from build123d import *

# Parameters (mm, degrees)
SKETCH1_R           = 4.2
BOSS_EXTRUDE1_DEPTH = 5
FILLET1_R           = 10
FILLET2_R           = 6
SKETCH2_W           = 42
SKETCH2_H           = 46
SKETCH2_R           = 11.5
SKETCH2_R_2         = 1.75
BOSS_EXTRUDE2_DEPTH = 4
CUT_EXTRUDE1_REACH  = 89.139
CUT_EXTRUDE1_START  = -1
SKETCH3_R           = 3
CUT_EXTRUDE2_REACH  = 90.34
SKETCH4_R           = 1.75
SKETCH5_R           = 2.1
CUT_EXTRUDE3_DEPTH  = 4
BOSS_EXTRUDE3_START = -2
BOSS_EXTRUDE3_DEPTH = 3
FILLET3_R           = 2
FILLET4_R           = 3
SKETCH7_R           = 1.75
CUT_EXTRUDE4_DEPTH  = 81.398748245
SKETCH8_R           = 2.1
CUT_EXTRUDE5_DEPTH  = 4
CHAMFER1_SIZE       = 0.5


with BuildPart() as part:
    # Sketch1 → Boss-Extrude1 (new, symmetric)
    with BuildSketch(Plane.XY):
        with BuildLine():
            Line((-52, 25), (52, 25))
            Line((52, 25), (52, 15.565713714))
            ThreePointArc((52, 15.565713714), (46, 1.282856857), (52, -13))
            Line((52, -13), (52, -25))
            Line((52, -25), (30, -25))
            ThreePointArc((30, -25), (0, -19.161984871), (-30, -25))
            Line((-30, -25), (-52, -25))
            Line((-52, -25), (-52, -13))
            ThreePointArc((-52, -13), (-46, 1.282856857), (-52, 15.565713714))
            Line((-52, 15.565713714), (-52, 25))
        make_face()
        with Locations((0, -11)):
            Circle(SKETCH1_R, mode=Mode.SUBTRACT)
        with Locations((-32, 7)):
            Circle(SKETCH1_R, mode=Mode.SUBTRACT)
        with Locations((32, 7)):
            Circle(SKETCH1_R, mode=Mode.SUBTRACT)
        with BuildLine():
            Line((-9.5, 21), (9.5, 21))
            ThreePointArc((9.5, 21), (10.560660172, 20.560660172), (11, 19.5))
            Line((11, 19.5), (11, 2.5))
            ThreePointArc((11, 2.5), (10.560660172, 1.439339828), (9.5, 1))
            Line((9.5, 1), (-9.5, 1))
            ThreePointArc((-9.5, 1), (-10.560660172, 1.439339828), (-11, 2.5))
            Line((-11, 2.5), (-11, 19.5))
            ThreePointArc((-11, 19.5), (-10.560660172, 20.560660172), (-9.5, 21))
        make_face(mode=Mode.SUBTRACT)
    extrude(amount=BOSS_EXTRUDE1_DEPTH, both=True)

    # Fillet1
    # the kernel refuses this fillet: 10 mm, written as the material it takes off along each edge
    with BuildSketch(Plane(origin=(52, 15.565713714, 14.292857857), x_dir=(-0.6589710561597435, -0.7521682970876347, 0), z_dir=(0, 0, -1))) as fillet1_piece_1:
        with BuildLine():
            CenterArc((3.793793334, 9.971172714), FILLET1_R, 228.778553177, 36.869897646)
            Line((-2.795917228, 2.449489743), (0, 0))
            ThreePointArc((0, 0), (1.517517334, 0.057654573), (3.035034667, 0))
        make_face()
    extrude(amount=28.585715715, mode=Mode.SUBTRACT)
    with BuildSketch(Plane(origin=(52, -13, 14.292857857), x_dir=(0, -1, 0), z_dir=(0, 0, -1)), Plane(origin=(-52, -13, -14.292857857), x_dir=(0, -1, 0), z_dir=(0, 0, 1))) as fillet1_piece_2:
        with BuildLine():
            CenterArc((3.717143143, 10), FILLET1_R, 233.130102354, 36.869897646)
            ThreePointArc((-2.282856857, 2), (-1.103435734, 1.043365942), (0, 0))
            Line((0, 0), (3.717143143, 0))
        make_face()
    extrude(amount=28.585715715, mode=Mode.SUBTRACT)
    with BuildSketch(Plane(origin=(52, -25, 30), x_dir=(-1, 0, 0), z_dir=(0, 0, -1))) as fillet1_piece_3:
        with BuildLine():
            CenterArc((FILLET1_R, FILLET1_R), FILLET1_R, 180, 90)
            Line((0, FILLET1_R), (0, 0))
            Line((0, 0), (FILLET1_R, 0))
        make_face()
    extrude(amount=60, mode=Mode.SUBTRACT)
    with BuildSketch(Plane(origin=(30, -25, 9.716697693), x_dir=(-0.931136532102541, 0.3646707536724787, 0), z_dir=(0, 0, -1))) as fillet1_piece_4:
        with BuildLine():
            CenterArc((1.889951723, 9.999382002), FILLET1_R, 248.612678269, 20.750330625)
            Line((-1.756755813, 0.688016681), (0, 0))
            ThreePointArc((0, 0), (0.889389046, 0.004943983), (1.778778093, 0))
        make_face()
    extrude(amount=19.433395387, mode=Mode.SUBTRACT)
    with BuildSketch(Plane(origin=(-30, -25, 9.716697693), x_dir=(-1, 0, 0), z_dir=(0, 0, -1))) as fillet1_piece_5:
        with BuildLine():
            CenterArc((1.886679077, 10), FILLET1_R, 249.249669375, 20.750330625)
            ThreePointArc((-1.656285265, 0.648668348), (-0.826339706, 0.328937697), (0, 0))
            Line((0, 0), (1.886679077, 0))
        make_face()
    extrude(amount=19.433395387, mode=Mode.SUBTRACT)
    with BuildSketch(Plane(origin=(-52, -25, -30), x_dir=(0, 1, 0), z_dir=(0, 0, 1))) as fillet1_piece_6:
        with BuildLine():
            CenterArc((FILLET1_R, -FILLET1_R), FILLET1_R, 90, 90)
            Line((0, -FILLET1_R), (0, 0))
            Line((0, 0), (FILLET1_R, 0))
        make_face()
    extrude(amount=60, mode=Mode.SUBTRACT)
    with BuildSketch(Plane(origin=(-52, 15.565713714, -14.292857857), x_dir=(0, 1, 0), z_dir=(0, 0, 1))) as fillet1_piece_7:
        with BuildLine():
            CenterArc((3.717143143, -10), FILLET1_R, 90, 36.869897646)
            ThreePointArc((-2.282856857, -2), (-1.103435734, -1.043365942), (0, 0))
            Line((0, 0), (3.717143143, 0))
        make_face()
    extrude(amount=28.585715715, mode=Mode.SUBTRACT)

    # Fillet2
    fillet2_edges = [part.edges().sort_by_distance(p)[0] for p in [
        (52, 25, 0),
        (-52, 25, 0),
    ]]
    fillet(fillet2_edges, radius=FILLET2_R)

    # Sketch2 → Boss-Extrude2 (add)
    with BuildSketch(Plane(origin=(0, 25, -30), x_dir=(-1, 0, 0), z_dir=(0, 1, 0))):
        with Locations((0, 2)):
            Rectangle(SKETCH2_W, SKETCH2_H)
        with Locations(Location((0, 1, 0), (0, 0, 90))):
            Circle(SKETCH2_R, mode=Mode.SUBTRACT)
        with Locations(Location((15.5, 16.5, 0), (0, 0, 90))):
            Circle(SKETCH2_R_2, mode=Mode.SUBTRACT)
        with Locations(Location((-15.5, 16.5, 0), (0, 0, 90))):
            Circle(SKETCH2_R_2, mode=Mode.SUBTRACT)
        with Locations(Location((-15.5, -14.5, 0), (0, 0, 90))):
            Circle(SKETCH2_R_2, mode=Mode.SUBTRACT)
        with Locations(Location((15.5, -14.5, 0), (0, 0, 90))):
            Circle(SKETCH2_R_2, mode=Mode.SUBTRACT)
    extrude(amount=-BOSS_EXTRUDE2_DEPTH)

    # Sketch3 → Cut-Extrude1 (cut, up to next)
    with BuildSketch(Plane.XZ.offset(-21).offset(CUT_EXTRUDE1_START), mode=Mode.PRIVATE) as cut_extrude1_sk1:
        with Locations(Location((-15.5, -44.5, 0), (0, 0, 270))):
            Circle(SKETCH3_R)
    cut_extrude1_tool1 = extrude(cut_extrude1_sk1.sketch, amount=CUT_EXTRUDE1_REACH, mode=Mode.PRIVATE) & part.part
    # Sketch3 → Cut-Extrude1 (cut, up to next)
    with BuildSketch(Plane.XZ.offset(-21).offset(CUT_EXTRUDE1_START), mode=Mode.PRIVATE) as cut_extrude1_sk2:
        with Locations(Location((15.5, -44.5, 0), (0, 0, 270))):
            Circle(SKETCH3_R)
    cut_extrude1_tool2 = extrude(cut_extrude1_sk2.sketch, amount=CUT_EXTRUDE1_REACH, mode=Mode.PRIVATE) & part.part
    # Sketch3 → Cut-Extrude1 (cut, up to next)
    with BuildSketch(Plane.XZ.offset(-21).offset(CUT_EXTRUDE1_START), mode=Mode.PRIVATE) as cut_extrude1_sk3:
        with Locations(Location((15.5, -13.5, 0), (0, 0, 270))):
            Circle(SKETCH3_R)
    cut_extrude1_tool3 = extrude(cut_extrude1_sk3.sketch, amount=CUT_EXTRUDE1_REACH, mode=Mode.PRIVATE) & part.part
    # Sketch3 → Cut-Extrude1 (cut, up to next)
    with BuildSketch(Plane.XZ.offset(-21).offset(CUT_EXTRUDE1_START), mode=Mode.PRIVATE) as cut_extrude1_sk4:
        with Locations(Location((-15.5, -13.5, 0), (0, 0, 270))):
            Circle(SKETCH3_R)
    cut_extrude1_tool4 = extrude(cut_extrude1_sk4.sketch, amount=CUT_EXTRUDE1_REACH, mode=Mode.PRIVATE) & part.part
    add(cut_extrude1_tool1.solids().sort_by_distance((-15.5, 22, -44.5))[0], mode=Mode.SUBTRACT)
    add(cut_extrude1_tool2.solids().sort_by_distance((15.5, 22, -44.5))[0], mode=Mode.SUBTRACT)
    add(cut_extrude1_tool3.solids().sort_by_distance((15.5, 22, -13.5))[0], mode=Mode.SUBTRACT)
    add(cut_extrude1_tool4.solids().sort_by_distance((-15.5, 22, -13.5))[0], mode=Mode.SUBTRACT)

    # Sketch4 → Cut-Extrude2 (cut, up to next)
    with BuildSketch(Plane(origin=(0, 25, 0), x_dir=(1, 0, 0), z_dir=(0, 1, 0)), mode=Mode.PRIVATE) as cut_extrude2_sk1:
        with Locations(Location((-32, 0, 0), (0, 0, 270))):
            Circle(SKETCH4_R)
    cut_extrude2_tool1 = extrude(cut_extrude2_sk1.sketch, amount=-CUT_EXTRUDE2_REACH, mode=Mode.PRIVATE) & part.part
    # Sketch4 → Cut-Extrude2 (cut, up to next)
    with BuildSketch(Plane(origin=(0, 25, 0), x_dir=(1, 0, 0), z_dir=(0, 1, 0)), mode=Mode.PRIVATE) as cut_extrude2_sk2:
        with Locations(Location((32, 0, 0), (0, 0, 270))):
            Circle(SKETCH4_R)
    cut_extrude2_tool2 = extrude(cut_extrude2_sk2.sketch, amount=-CUT_EXTRUDE2_REACH, mode=Mode.PRIVATE) & part.part
    add(cut_extrude2_tool1.solids().sort_by_distance((-32, 25, 0))[0], mode=Mode.SUBTRACT)
    add(cut_extrude2_tool2.solids().sort_by_distance((32, 25, 0))[0], mode=Mode.SUBTRACT)

    # Sketch5 → Cut-Extrude3 (cut)
    with BuildSketch(Plane(origin=(0, 25, 0), x_dir=(1, 0, 0), z_dir=(0, 1, 0))):
        with Locations(Location((-32, 0, 0), (0, 0, 270))):
            Circle(SKETCH5_R)
        with Locations(Location((32, 0, 0), (0, 0, 270))):
            Circle(SKETCH5_R)
    extrude(amount=-CUT_EXTRUDE3_DEPTH, mode=Mode.SUBTRACT)

    # Sketch6 → Boss-Extrude3 (add)
    with BuildSketch(Plane(origin=(21, 0, 0), x_dir=(0, 0, -1), z_dir=(1, 0, 0)).offset(BOSS_EXTRUDE3_START)):
        Polygon((51, 25), (5, 25), (5, 5), (51, 21), align=None)
    boss_extrude3 = extrude(amount=BOSS_EXTRUDE3_DEPTH)

    # Mirror1: Boss-Extrude3 across plane
    add(boss_extrude3.mirror(Plane(origin=(0, 0, 0), x_dir=(0, 0, 1), z_dir=(1, 0, 0))))

    # Fillet3
    fillet3_edges = [part.edges().sort_by_distance(p)[0] for p in [
        (-14.25, 21, -5),
        (14.25, 21, -5),
    ]]
    fillet(fillet3_edges, radius=FILLET3_R)

    # Fillet4
    fillet4_edges = [part.edges().sort_by_distance(p)[0] for p in [
        (22, 15, -5),
        (-22, 15, -5),
        (-22, 23, -51),
        (22, 23, -51),
    ]]
    fillet(fillet4_edges, radius=FILLET4_R)

    # Sketch7 → Cut-Extrude4 (cut, through all)
    with BuildSketch(Plane.XY.offset(5)):
        with Locations((-20, -9)):
            Circle(SKETCH7_R)
        with Locations((20, -9)):
            Circle(SKETCH7_R)
    extrude(amount=-CUT_EXTRUDE4_DEPTH, mode=Mode.SUBTRACT)

    # Sketch8 → Cut-Extrude5 (cut)
    with BuildSketch(Plane.XY.offset(5)):
        with Locations((-20, -9)):
            Circle(SKETCH8_R)
        with Locations((20, -9)):
            Circle(SKETCH8_R)
    extrude(amount=-CUT_EXTRUDE5_DEPTH, mode=Mode.SUBTRACT)

    # Chamfer1
    # the kernel refuses this chamfer: 0.5 mm, written as the material it takes off along each edge
    with BuildSketch(Plane(origin=(-32, 21, 0), x_dir=(0, 0, 1), z_dir=(-1, 0, 0))) as chamfer1_piece_1_section:
        Polygon((1.75, -CHAMFER1_SIZE), (1.75 + CHAMFER1_SIZE, 0), (1.75, 0), align=None)
    chamfer1_piece_1 = revolve(axis=Axis((-32, 21, 0), (0, 1, 0)), mode=Mode.PRIVATE)
    chamfer1_piece_1 = chamfer1_piece_1 & Plane(origin=(-32, 20.675956313, 0), x_dir=(0, 0, 1), z_dir=(0, 1, 0)) * Cylinder(2.1, 9, mode=Mode.PRIVATE)
    add(chamfer1_piece_1, mode=Mode.SUBTRACT)
    with BuildSketch(Plane(origin=(32, 21, 0), x_dir=(0, 0, 1), z_dir=(-1, 0, 0))) as chamfer1_piece_2_section:
        Polygon((1.75, -CHAMFER1_SIZE), (1.75 + CHAMFER1_SIZE, 0), (1.75, 0), align=None)
    chamfer1_piece_2 = revolve(axis=Axis((32, 21, 0), (0, 1, 0)), mode=Mode.PRIVATE)
    chamfer1_piece_2 = chamfer1_piece_2 & Plane(origin=(32, 20.675956313, 0), x_dir=(0, 0, 1), z_dir=(0, 1, 0)) * Cylinder(2.1, 10, mode=Mode.PRIVATE)
    add(chamfer1_piece_2, mode=Mode.SUBTRACT)
    with BuildSketch(Plane(origin=(-20, -9, 1), x_dir=(1, 0, 0), z_dir=(0, -1, 0))) as chamfer1_piece_3_section:
        Polygon((1.75, -CHAMFER1_SIZE), (1.75 + CHAMFER1_SIZE, 0), (1.75, 0), align=None)
    chamfer1_piece_3 = revolve(axis=Axis((-20, -9, 1), (0, 0, 1)), mode=Mode.PRIVATE)
    chamfer1_piece_3 = chamfer1_piece_3 & Plane(origin=(-20, -9, 0.675956313), x_dir=(1, 0, 0), z_dir=(0, 0, 1)) * Cylinder(2.1, 9, mode=Mode.PRIVATE)
    add(chamfer1_piece_3, mode=Mode.SUBTRACT)
    with BuildSketch(Plane(origin=(20, -9, 1), x_dir=(1, 0, 0), z_dir=(0, -1, 0))) as chamfer1_piece_4_section:
        Polygon((1.75, -CHAMFER1_SIZE), (1.75 + CHAMFER1_SIZE, 0), (1.75, 0), align=None)
    chamfer1_piece_4 = revolve(axis=Axis((20, -9, 1), (0, 0, 1)), mode=Mode.PRIVATE)
    chamfer1_piece_4 = chamfer1_piece_4 & Plane(origin=(20, -9, 0.675956313), x_dir=(1, 0, 0), z_dir=(0, 0, 1)) * Cylinder(2.1, 9, mode=Mode.PRIVATE)
    add(chamfer1_piece_4, mode=Mode.SUBTRACT)


solid = part.part
The model under review builds one solid part; all positions refer to its coordinate system, in mm. A direction names the side the tool comes from. Round coordinates to 2 decimals unless told otherwise and drop trailing zeros. Write each loop counter-clockwise with the first axis right and the second up, starting at its lowest first coordinate (ties: lowest second). Pieces come first, ordered by that corner, then holes. Notation, with made-up numbers: M 27,20.25 L 52,20.25 A18 ccw 52,31.25 Z; hole C 84.25,72 d10. An arc over 180 degrees is marked long. Answer as CSV lines item,"result". Start each with the question number.
Q1. Wall thickness on line 1 along X through (y, z) = (23.95, -13.5); line 2 along X through (y, z) = (13.75, 0); line 3 along Z through (x, y) = (15.5, 21.2): over which ranges is each line inside the solid? List them lowest first.
Q2. The part is to be moulded in two halves that separate along Y. For faces 1 (the face through (-51.38, 15.82, -0.07)), 2 (the face through (22, 18, -23)), 3 (the face through (-17, 22, -15)), say which applies: +Y half, -Y half, draft (parallel to the pull), parting line (faces both ways), or undercut.
Q3. Consider section B-B, the plane y = -9. Give the boundary of the cut face in (x, z).
Q4. Consider section D-D, the plane x = -15.5. Give the boundary of the cut face in (y, z).
Q5. Tool access review of faces 4 (the face through (14.18, 20.43, -5.6)), 5 (the face through (22.9, 14.86, -5.86)): name each direction out of +Z, -Z, +X, -X, +Y, -Y from which nothing blocks a thin tool from reaching the whole face with its end or side.
Q6. Consider section A-A, the plane x = 0. Give the boundary of the cut face in (y, z), then the cut area to 3 significant figures.
Q7. Consider section C-C, the plane z = -23. Give the boundary of the cut face in (x, y), then the cut area to 3 significant figures.
Q8. Clearance check with flat-ended pins moving along their axes: P1, Ø13, axis at y = 11.5, z = -31, coming from the +X side; P2, Ø11, axis at x = 0, y = -11, coming from the -Z side; P3, Ø3, axis at y = 10.5, z = -18.5, coming from the -X side. State where each tip first meets the part, or that it passes through.
Result set:
1,line 1,"x = -22 to -17.25, -13.75 to 13.75, 17.25 to 22"
1,line 2,"x = -50.33 to -33.75, -30.25 to -11, 11 to 30.25, 33.75 to 50.33"
1,line 3,"z = -51 to -47.5, -41.5 to -16.5, -10.5 to 5"
2,face 1,"undercut"
2,face 2,"draft"
2,face 3,"-Y half"
3,outline,"M -48.85,-5 L -21.75,-5 L -21.75,0.5 L -22.1,0.85 L -22.1,5 L -48.85,5 Z; M -18.25,-5 L -3.69,-5 L -3.69,5 L -17.9,5 L -17.9,0.85 L -18.25,0.5 Z; M 3.69,-5 L 18.25,-5 L 18.25,0.5 L 17.9,0.85 L 17.9,5 L 3.69,5 Z; M 21.75,-5 L 48.85,-5 L 48.85,5 L 22.1,5 L 22.1,0.85 L 21.75,0.5 Z"
4,outline,"M -20.68,-5 L 19,-5 A2 cw 21,-7 L 21,-10.5 L 22,-10.5 L 22,-11.75 L 25,-11.75 L 25,5 L -20.68,5 Z; M 21,-51 L 25,-51 L 25,-46.25 L 22,-46.25 L 22,-47.5 L 21,-47.5 Z; M 21,-41.5 L 22,-41.5 L 22,-42.75 L 25,-42.75 L 25,-15.25 L 22,-15.25 L 22,-16.5 L 21,-16.5 Z"
5,face 4,"-Z, -Y"
5,face 5,"-Z, +X, +Y, -Y"
6,outline,"M -19.16,-5 L -15.2,-5 L -15.2,5 L -19.16,5 Z; M -6.8,-5 L 1,-5 L 1,5 L -6.8,5 Z; M 21,-51 L 25,-51 L 25,-40.5 L 21,-40.5 Z; M 21,-17.5 L 25,-17.5 L 25,5 L 21,5 Z"
6,area,"250 mm²"
7,outline,"M -22,11.26 L -19,11.26 L -19,21 L -9.81,21 L -9.81,25 L -22,25 Z; M 9.81,21 L 19,21 L 19,11.26 L 22,11.26 L 22,25 L 9.81,25 Z"
7,area,"156 mm²"
8,P1,"stops at x = 22"
8,P2,"stops at z = -5"
8,P3,"stops at x = -22"
